from build123d import *

# Parameters (mm, degrees)
SKETCH_1_W          = 2200
SKETCH_1_H          = 1250
SKETCH_1_R          = 550
EXTRUDE_1_DEPTH     = 10
SKETCH_2_R          = 4.05
CUT_EXTRUDE_1_DEPTH = 10
CUT_EXTRUDE_2_DEPTH = 10


with BuildPart() as part:
    # 草图1 → 凸台-拉伸1 (new body)
    with BuildSketch(Plane(origin=(0, 0, 0), x_dir=(1, 0, 0), z_dir=(0, 1, 0))):
        Rectangle(SKETCH_1_W, SKETCH_1_H)
        with Locations(Location((480, 0, 0), (0, 0, 270))):
            Circle(SKETCH_1_R, mode=Mode.SUBTRACT)
    extrude(amount=EXTRUDE_1_DEPTH)

    # 草图2 → 切除-拉伸1 (cut)
    with BuildSketch(Plane(origin=(0, 10, 0), x_dir=(1, 0, 0), z_dir=(0, 1, 0))):
        with Locations(Location((-1080, 565, 0), (0, 0, 270))):
            Circle(SKETCH_2_R)
        with Locations(Location((-1080, -565, 0), (0, 0, 270))):
            Circle(SKETCH_2_R)
        with Locations(Location((1080, -565, 0), (0, 0, 270))):
            Circle(SKETCH_2_R)
        with Locations(Location((1080, 565, 0), (0, 0, 270))):
            Circle(SKETCH_2_R)
    extrude(amount=-CUT_EXTRUDE_1_DEPTH, mode=Mode.SUBTRACT)

    # 草图3 → 切除-拉伸2 (cut)
    with BuildSketch(Plane(origin=(0, 10, 0), x_dir=(1, 0, 0), z_dir=(0, 1, 0))):
        Polygon((-1100, 625), (-1060, 625), (-1060, 620), (-1095, 620), (-1095, 585), (-1100, 585), align=None)
        Polygon((-1100, -585), (-1100, -625), (-1060, -625), (-1060, -620), (-1095, -620), (-1095, -585), align=None)
        Polygon((1100, -625), (1060, -625), (1060, -620), (1095, -620), (1095, -585), (1100, -585), align=None)
        Polygon((1100, 585), (1100, 625), (1060, 625), (1060, 620), (1095, 620), (1095, 585), align=None)
    extrude(amount=-CUT_EXTRUDE_2_DEPTH, mode=Mode.SUBTRACT)


solid = part.part
The model under review builds one solid part; all positions refer to its coordinate system, in mm. Round coordinates to 2 decimals unless told otherwise and drop trailing zeros. Loops run counter-clockwise (first coordinate to the right, second up) from the corner with the lowest first, then second, coordinate; pieces in that order, holes last. Notation, with made-up numbers: (-5, 2) -> (47, 2) arc R32 cw to (47, 31) -> close; hole circle Ø1 at (69.5, 22). An arc over 180 degrees is marked (long way). One line per question, with ' | ' between items. Start each with the question number.
Item 1: Add section B-B, the plane z = 0. Write out the cut boundary in (x, y), then the cut area to 3 significant figures.
Item 2: Draft analysis for pull direction X (two halves, no side actions). For faces 1 (the face through (145.33, 4.93, -436.46)), 2 (the face through (-260, 10, -9)), state which applies: +X half, -X half, draft (parallel to the pull), parting line (faces both ways), or undercut.
Item 3: Add section A-A, the plane x = 480. Write out the cut boundary in (y, z).
Item 4: For pin 1 (3 mm diameter, centred on x = 1079.5, y = 3.5, fed in from +Z); pin 2 (4 mm diameter, centred on x = -1097.5, y = 3, fed in from +Z); pin 3 (5.5 mm diameter, centred on x = -1096.5, y = 4.5, fed in from -Z), all flat-tipped, find the tip position at first contact; note any pin that passes through.
Item 5: Wall thickness on line 1 along Z through (x, y) = (-1080, 6); line 2 along X through (y, z) = (2, -565); line 3 along X through (y, z) = (1.5, 563): over which ranges is each line inside the solid? List them lowest first. Write a range as [from, to].
Item 6: Add section C-C, the plane y = 4. Write out the cut boundary in (x, z).
Return value:
1) outline: (-1100, 0) -> (-70, 0) -> (-70, 10) -> (-1100, 10) -> close; (1030, 0) -> (1100, 0) -> (1100, 10) -> (1030, 10) -> close | area: 11,000 mm2
2) face 1: undercut | face 2: draft
3) outline: (0, -625) -> (10, -625) -> (10, -550) -> (0, -550) -> close; (0, 550) -> (10, 550) -> (10, 625) -> (0, 625) -> close
4) pin 1: stops at z = 620 | pin 2: stops at z = 585 | pin 3: stops at z = -620
5) line 1: z = [-620, -569.05], [-560.95, 560.95], [569.05, 620] | line 2: x = [-1100, -1084.05], [-1075.95, 1075.95], [1084.05, 1100] | line 3: x = [-1100, -1083.52], [-1076.48, 1076.48], [1083.52, 1100]
6) outline: (-1100, -585) -> (-1095, -585) -> (-1095, -620) -> (-1060, -620) -> (-1060, -625) -> (1060, -625) -> (1060, -620) -> (1095, -620) -> (1095, -585) -> (1100, -585) -> (1100, 585) -> (1095, 585) -> (1095, 620) -> (1060, 620) -> (1060, 625) -> (-1060, 625) -> (-1060, 620) -> (-1095, 620) -> (-1095, 585) -> (-1100, 585) -> close; hole circle Ø8.1 at (-1080, -565); hole circle Ø8.1 at (-1080, 565); hole circle Ø1100 at (480, 0); hole circle Ø8.1 at (1080, -565); hole circle Ø8.1 at (1080, 565)
